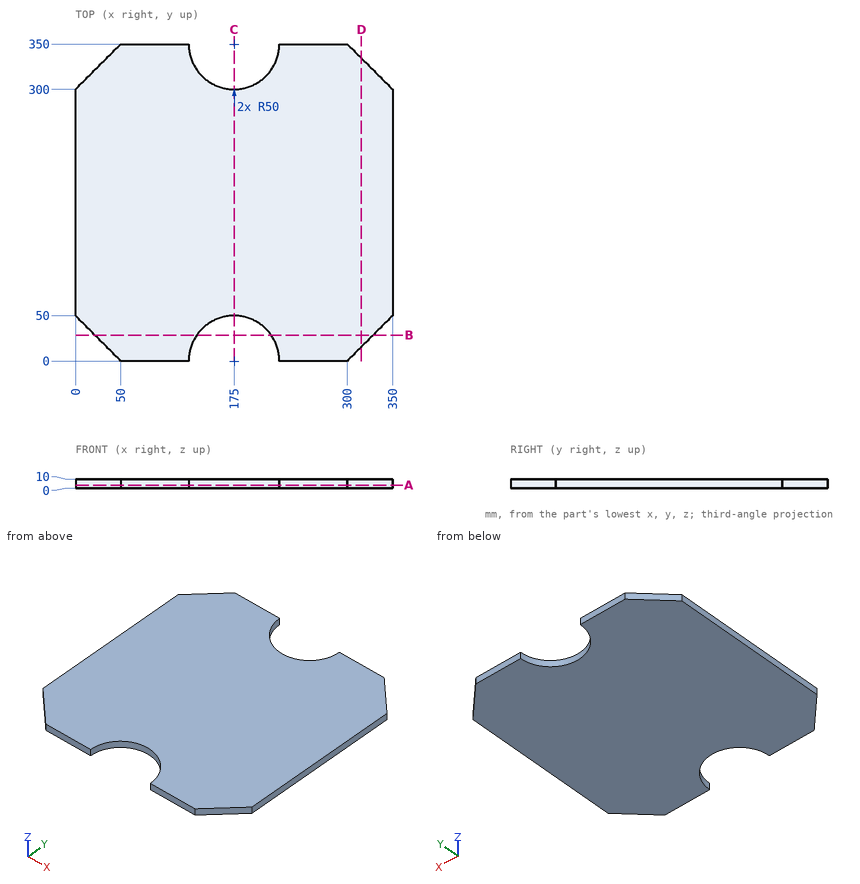
Geometry check sheet. Reference: drawing and pictorial views, mm from the part's lowest x, y, z. Round coordinates to 2 decimals unless told otherwise and drop trailing zeros. Loops run counter-clockwise (first coordinate to the right, second up) from the corner with the lowest first, then second, coordinate; pieces in that order, holes last. Notation, with made-up numbers: (8.25, -17) -> (60.25, -17) arc R17 ccw to (60.25, -5) -> close; hole circle Ø5 at (-11.5, 7.5). An arc over 180 degrees is marked (long way). Answer as a JSON object with one key per item and string values.
Q1. Section check B-B (y = 28.5). Record the boundary of the cut face in (x, z).
Data:
{"outline": "(21.5, 0) -> (133.92, 0) -> (133.92, 10) -> (21.5, 10) -> close; (216.08, 0) -> (328.5, 0) -> (328.5, 10) -> (216.08, 10) -> close"}
Q2. Scan lines: line 1 (X direction, y = 328.5, z = 5.5); line 2 (X direction, y = 36.5, z = 9.75); line 3 (Y direction, x = 196, z = 5). Record each from-to range of solid material in increasing order. Write a range as from..to.
Data:
{"line 1": "x = 28.5..129.86, 220.14..321.5", "line 2": "x = 13.5..140.83, 209.17..336.5", "line 3": "y = 45.38..304.62"}
Q3. Section check D-D (x = 315.5). Record the boundary of the cut face in (y, z).
Data:
{"outline": "(15.5, 0) -> (334.5, 0) -> (334.5, 10) -> (15.5, 10) -> close"}
Q4. Section check A-A (z = 3.25). Record the boundary of the cut face in (x, y), then the cut area to 3 significant figures.
Data:
{"outline": "(0, 50) -> (50, 0) -> (125, 0) arc R50 cw to (225, 0) -> (300, 0) -> (350, 50) -> (350, 300) -> (300, 350) -> (225, 350) arc R50 cw to (125, 350) -> (50, 350) -> (0, 300) -> close", "area": "110,000 mm2"}
Q5. Section check C-C (x = 175). Record the boundary of the cut face in (y, z).
Data:
{"outline": "(50, 0) -> (300, 0) -> (300, 10) -> (50, 10) -> close"}
